from build123d import *

# Parameters (mm, degrees)
F1_DEPTH = 25


with BuildPart() as f1:
    # F0 (on Top) → F1 (new body)
    with BuildSketch(Plane.XY):
        with BuildLine():
            ThreePointArc((7.679492, -4), (19.803848, 3), (19.803848, 17))
            Line((19.803848, 17), (12.124356, 30.30127))
            ThreePointArc((12.124356, 30.30127), (0, 37.30127), (-12.124356, 30.30127))
            Line((-12.124356, 30.30127), (-19.803848, 17))
            ThreePointArc((-19.803848, 17), (-19.803848, 3), (-7.679492, -4))
            Line((-7.679492, -4), (0, -4))
            Line((0, -4), (7.679492, -4))
        make_face()
        with BuildLine():
            Line((7.679492, 0), (0, 0))
            Line((0, 0), (-7.679492, 0))
            ThreePointArc((-7.679492, 0), (-16.339746, 5), (-16.339746, 15))
            Line((-16.339746, 15), (-8.660254, 28.30127))
            ThreePointArc((-8.660254, 28.30127), (0, 33.30127), (8.660254, 28.30127))
            Line((8.660254, 28.30127), (16.339746, 15))
            ThreePointArc((16.339746, 15), (16.339746, 5), (7.679492, 0))
        make_face(mode=Mode.SUBTRACT)
    extrude(amount=F1_DEPTH)


solid = f1.part
Part model, mm, in its own coordinate system. A direction names the side the tool comes from. Coordinates: 2 decimals unless noted, no trailing zeros. Loops run counter-clockwise (first coordinate to the right, second up) from the corner with the lowest first, then second, coordinate; pieces in that order, holes last. Notation, with made-up numbers: M -14,26.25 L -2,26.25 A24 ccw -2,43.25 Z; hole C 69.5,43 d11. An arc over 180 degrees is marked long. Use a Markdown table: item, result. Add a question column.
Q1. Cut at C-C (z = 12). Write the cut outline in (x, y), and give its area (3 significant figures).
Q2. Mould opens along Y. For faces 1 (the cylindrical face through (-16.266, 4.874, 12.325)), 2 (the cylindrical face through (-19.905, 3.178, 12.325)), 3 (the cylindrical face through (0.2, 37.3, 12.3)) say: +Y half, -Y half, draft (parallel to the pull), parting line (faces both ways), or undercut.
Q3. Which spindle directions (+Z, -Z, +X, -X, +Y, -Y) get a long thin tool onto all of the face, cutting with end or side? Do faces 4 (the flat face through (-11.3, 24.4, 25)), 5 (the cylindrical face through (16.412, 5.127, 12.325)). Say none if no direction does.
Q4. Cut at B-B (y = 23). Write the cut outline in (x, z).
Q5. Probe L1, parallel to Y at x = 11, z = 15.5; L2, parallel to X at y = 21, z = 23.25; L3, parallel to X at y = 10, z = 4.25. List the from-to ranges inside material, lowest first.
Q6. Cut at D-D (y = -1). Write the cut outline in (x, z), and give its area (3 significant figures).
Q7. Pin check, flat tips, straight feed: P1, Ø12, axis at x = 10.5, z = 11.5, coming from the +Y side; P2, Ø5, axis at x = 10.5, z = 8, coming from the -Y side; P3, Ø8, axis at x = 16.5, z = 16.5, coming from the +Y side. Stop position of each tip, or through.
Q8. Cut at A-A (x = 11). Write the cut outline in (y, z).
Worked out:
| question | item | result |
|---|---|---|
| 1 | outline | M -19.8,17 A14 ccw -7.68,-4 L 7.68,-4 A14 ccw 19.8,17 L 12.12,30.3 A14 ccw -12.12,30.3 Z; hole M -16.34,15 A10 ccw -7.68,0 L 7.68,0 A10 ccw 16.34,15 L 8.66,28.3 A10 ccw -8.66,28.3 Z |
| 1 | area | 486 mm2 |
| 2 | face 1 | undercut |
| 2 | face 2 | parting line |
| 2 | face 3 | +Y half |
| 3 | face 4 | +Z, +X, -X, +Y, -Y |
| 3 | face 5 | +Z, -Z |
| 4 | outline | M -16.34,0 L -11.72,0 L -11.72,25 L -16.34,25 Z; M 11.72,0 L 16.34,0 L 16.34,25 L 11.72,25 Z |
| 5 | L1 | y = -3.6 to 0.57, 24.25 to 31.96 |
| 5 | L2 | x = -17.49 to -12.88, 12.88 to 17.49 |
| 5 | L3 | x = -21.68 to -17.68, 17.68 to 21.68 |
| 6 | outline | M -16.34,0 L 16.34,0 L 16.34,25 L -16.34,25 Z |
| 6 | area | 817 mm2 |
| 7 | P1 | stops at y = 36.56 |
| 7 | P2 | stops at y = -4 |
| 7 | P3 | stops at y = 29.65 |
| 8 | outline | M -3.6,0 L 0.57,0 L 0.57,25 L -3.6,25 Z; M 24.25,0 L 31.96,0 L 31.96,25 L 24.25,25 Z |
